```python
from build123d import *

# Parameters (mm, degrees)
SKETCH1_W           = 80
SKETCH1_H           = 65
SKETCH1_R           = 5
BOSS_EXTRUDE1_DEPTH = 5
SCALE2_SCALE        = 0.1


with BuildPart() as part:
    # Sketch1 → Boss-Extrude1 (new body)
    with BuildSketch(Plane(origin=(0, 0, 0), x_dir=(1, 0, 0), z_dir=(0, 1, 0))):
        with Locations((0, 7.5)):
            Rectangle(SKETCH1_W, SKETCH1_H)
        with Locations(Location((-30, 30, 0), (0, 0, 270))):
            Circle(SKETCH1_R, mode=Mode.SUBTRACT)
        with Locations(Location((30, 30, 0), (0, 0, 270))):
            Circle(SKETCH1_R, mode=Mode.SUBTRACT)
    extrude(amount=BOSS_EXTRUDE1_DEPTH)


with BuildPart() as part_1:
    # Scale2: scaled about (0, 2.5, -6.799157734)
    add(part.part.scale(SCALE2_SCALE).moved(Location((0, 2.25, -6.119241961))))


solid = part_1.part
```
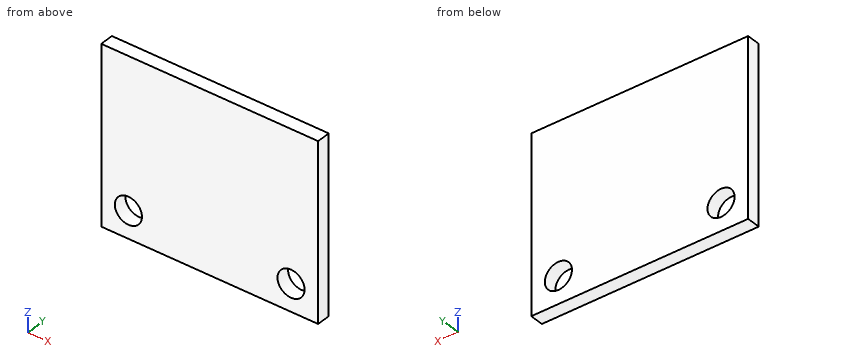
Could you check a few things on this model? Use its own coordinates, in mm. Give positions to 0.01 mm unless a question says otherwise; leave off trailing zeros. Write each loop counter-clockwise with the first axis right and the second up, starting at its lowest first coordinate (ties: lowest second). Pieces come first, ordered by that corner, then holes. Notation, with made-up numbers: (52, 31) -> (103, 31) arc R21 cw to (103, 50) -> close; hole circle Ø7 at (-2.75, 81). An arc over 180 degrees is marked (long way). Write each question's results on one line, items separated by ' | '.
1. I want a section at A-A, the plane x = -3. Write out the boundary of the cut face in (y, z), then the cut area to 3 significant figures.
Check sheet entries:
outline: (2.25, -10.12) -> (2.75, -10.12) -> (2.75, -9.62) -> (2.25, -9.62) -> close; (2.25, -8.62) -> (2.75, -8.62) -> (2.75, -3.62) -> (2.25, -3.62) -> close | area: 2.75 mm²
2. I need wall thicknesses on L1, parallel to X at y = 2.45, z = -9.25; L2, parallel to X at y = 2.3, z = -9.5; L3, parallel to Z at x = -2.75, y = 2.55. Which ranges of each line are inside material? Lowest first, please.
Check sheet entries:
L1: x = -4 to -3.48, -2.52 to 2.52, 3.48 to 4 | L2: x = -4 to -3.32, -2.68 to 2.68, 3.32 to 4 | L3: z = -10.12 to -9.55, -8.69 to -3.62
3. I want a section at C-C, the plane z = -9.5. Write out the boundary of the cut face in (x, y), then the cut area to 3 significant figures.
Check sheet entries:
outline: (-4, 2.25) -> (-3.32, 2.25) -> (-3.32, 2.75) -> (-4, 2.75) -> close; (-2.68, 2.25) -> (2.68, 2.25) -> (2.68, 2.75) -> (-2.68, 2.75) -> close; (3.32, 2.25) -> (4, 2.25) -> (4, 2.75) -> (3.32, 2.75) -> close | area: 3.35 mm²
4. I want a section at B-B, the plane y = 2.4. Write out the boundary of the cut face in (x, z), then the cut area to 3 significant figures.
Check sheet entries:
outline: (-4, -10.12) -> (4, -10.12) -> (4, -3.62) -> (-4, -3.62) -> close; hole circle Ø1 at (-3, -9.12); hole circle Ø1 at (3, -9.12) | area: 50.4 mm²
